Read the model definition and answer for the solid it produces. Units are mm, in the model's axes. Face numbers are marked on the shaded views. A direction names the side the tool comes from. Give positions to 0.01 mm unless a question says otherwise; leave off trailing zeros. Write each loop counter-clockwise with the first axis right and the second up, starting at its lowest first coordinate (ties: lowest second). Pieces come first, ordered by that corner, then holes. Notation, with made-up numbers: (-16, 70) -> (1, 70) arc R9 ccw to (1, 80) -> close; hole circle Ø1 at (34, 2.25). An arc over 180 degrees is marked (long way). Use a Markdown table: item, result.
from build123d import *

# Parameters (mm, degrees)
PAD002_DEPTH    = 5.55
POCKET001_DEPTH = 0.5
POCKET002_DEPTH = 0.5
PAD003_DEPTH    = 2.5
PAD001_DEPTH    = 9
SKETCH_R        = 9
PAD_DEPTH       = 11.8
SKETCH001_R     = 11.05
POCKET_DEPTH    = 10
SKETCH010_R     = 1.55
POCKET003_DEPTH = 5
FILLET_R        = 1.8
SKETCH012_W     = 10.3286741025
SKETCH012_H     = 11.8
PAD004_DEPTH    = 2.4
SKETCH011_R     = 2.1
POCKET004_DEPTH = 6.4010000001
POCKET005_DEPTH = 4
FILLET001_R     = 2
FILLET002_R     = 2
FILLET003_R     = 2


with BuildPart() as pad003:
    # Sketch004 → Pad002 (new body)
    with BuildSketch(Plane.XY.offset(2.225)):
        Polygon((-11.1717282118, -2.7499991288), (-7.9674332118, -8.3000008712), (-8.4004459137, -8.5500008712), (-11.6047409137, -2.9999991288), align=None)
    extrude(amount=PAD002_DEPTH)

    # Sketch006 → Pocket001 (cut)
    with BuildSketch(Plane(origin=(-9.5695807118, -5.525, 2.225), x_dir=(-0.5, 0.8660254038, 0), z_dir=(0.8660254038, 0.5, 0))):
        Polygon((-3.204295, 2.7750019602), (-1.6021491347, 5.55), (-3.204295, 5.55), align=None)
        Polygon((1.6021478772, 0), (3.204295, 0), (3.204295, 2.7750019602), align=None)
    extrude(amount=-POCKET001_DEPTH, mode=Mode.SUBTRACT)

    # Sketch008 → Pocket002 (cut)
    with BuildSketch(Plane(origin=(-9.5695807118, -5.525, 2.225), x_dir=(-0.5, 0.8660254038, 0), z_dir=(0.8660254038, 0.5, 0))):
        Polygon((1.6021478772, 5.5500030493), (3.204295, 5.5500030493), (3.204295, 2.7750019602), align=None)
        Polygon((-1.6021478772, 0), (-3.2042957545, 0), (-3.2042957545, 2.7750015246), align=None)
    extrude(amount=-POCKET002_DEPTH, mode=Mode.SUBTRACT)

    # Sketch009 → Pad003 (new body, symmetric)
    with BuildSketch(Plane(origin=(-9.5695807118, -5.525, 2.225), x_dir=(-0.5, 0.8660254038, 0), z_dir=(0.8660254038, 0.5, 0))):
        Polygon((1.6021491347, -7.4054e-06), (3.2042982695, 2.7749962973), (1.6021491347, 5.55), (-1.6021491347, 5.55), (-3.2042982695, 2.7749962973), (-1.6021491347, -7.4054e-06), align=None)
    extrude(amount=PAD003_DEPTH, both=True)


with BuildPart() as pad001:
    # Sketch003 → Pad001 (new body)
    with BuildSketch(Plane.XY):
        with BuildLine():
            ThreePointArc((-10.9554657182, -1.442314424), (-9.5695807118, -5.525), (-6.7268137905, -8.7665544102))
            Line((-10.3793823646, -13.526674452), (-6.7268137905, -8.7665544102))
            ThreePointArc((-16.9041348864, -2.2254715773), (-14.7657331345, -8.525), (-10.3793823646, -13.526674452))
            Line((-10.9554657182, -1.442314424), (-16.9041348864, -2.2254715773))
        make_face()
    extrude(amount=PAD001_DEPTH)


with BuildPart() as fillet003:
    # Sketch → Pad (new body)
    with BuildSketch(Plane.XY):
        with BuildLine():
            Line((-23, 11.5), (23, 11.5))
            Line((23, 11.5), (23, 7.5))
            Line((23, 7.5), (15, 7.5))
            Line((12.6713258975, 7.5), (15, 7.5))
            Line((12.6713258975, 4.8), (12.6713258975, 7.5))
            ThreePointArc((-12.6713258975, 4.8), (0, -13.55), (12.6713258975, 4.8))
            Line((-12.6713258975, 7.5), (-12.6713258975, 4.8))
            Line((-15, 7.5), (-12.6713258975, 7.5))
            Line((-15, 7.5), (-23, 7.5))
            Line((-23, 7.5), (-23, 11.5))
        make_face()
        Circle(SKETCH_R, mode=Mode.SUBTRACT)
    extrude(amount=PAD_DEPTH)

    # Sketch001 → Pocket (cut)
    with BuildSketch(Plane.XY.offset(11.8)):
        Circle(SKETCH001_R)
    extrude(amount=-POCKET_DEPTH, mode=Mode.SUBTRACT)

    # Fusion: union Pad001
    add(pad001.part)

    # Cut: cut Pad003
    add(pad003.part, mode=Mode.SUBTRACT)

    # Sketch010 → Pocket003 (cut)
    with BuildSketch(Plane(origin=(-11.7346442213, -6.775, 0), x_dir=(-0.5, 0.8660254038, 0), z_dir=(0.8660254038, 0.5, 0))):
        with Locations((0, 4.9999962973)):
            Circle(SKETCH010_R)
    extrude(amount=-POCKET003_DEPTH, mode=Mode.SUBTRACT)

    # Fillet
    fillet_edges = [fillet003.edges().sort_by_distance(p)[0] for p in [
        (-12.671326, 4.8, 5.9),
        (12.671326, 4.8, 5.9),
    ]]
    fillet(fillet_edges, radius=FILLET_R)

    # Sketch012 → Pad004 (new body)
    with BuildSketch(Plane.XZ.offset(-7.5)):
        with Locations((-17.8356629487, 5.9)):
            Rectangle(SKETCH012_W, SKETCH012_H)
        with Locations((17.8356629487, 5.9)):
            Rectangle(SKETCH012_W, SKETCH012_H)
    extrude(amount=PAD004_DEPTH)

    # Sketch011 → Pocket004 (cut, through all)
    with BuildSketch(Plane.XZ.offset(-5.1)):
        with Locations((-18.5, 5.9)):
            Circle(SKETCH011_R)
        with Locations((18.5, 5.9)):
            Circle(SKETCH011_R)
    extrude(amount=-POCKET004_DEPTH, mode=Mode.SUBTRACT)

    # Sketch013 → Pocket005 (cut)
    with BuildSketch(Plane.XZ.offset(-5.1)):
        Polygon((-14.4296806022, 5.9), (-16.4648403011, 9.425), (-20.5351596989, 9.425), (-22.5703193978, 5.9), (-20.5351596989, 2.375), (-16.4648403011, 2.375), align=None)
        Polygon((22.5703193978, 5.9), (20.5351596989, 9.425), (16.4648403011, 9.425), (14.4296806022, 5.9), (16.4648403011, 2.375), (20.5351596989, 2.375), align=None)
    extrude(amount=-POCKET005_DEPTH, mode=Mode.SUBTRACT)

    # Fillet001
    fillet001_edges = [fillet003.edges().sort_by_distance(p)[0] for p in [
        (-23, 6.3, 0),
        (-23, 9.5, 0),
        (-23, 9.5, 11.8),
        (-23, 6.3, 11.8),
        (23, 6.3, 0),
        (23, 9.5, 0),
        (23, 9.5, 11.8),
        (23, 6.3, 11.8),
    ]]
    fillet(fillet001_edges, radius=FILLET001_R)

    # Fillet002
    fillet002_edges = [fillet003.edges().sort_by_distance(p)[0] for p in [
        (-8.248717, -10.749938, 4.5),
        (-13.434078, -1.76863, 4.5),
    ]]
    fillet(fillet002_edges, radius=FILLET002_R)

    # Fillet003
    fillet003_edges = [fillet003.edges().sort_by_distance(p)[0] for p in [
        (-10.379382, -13.526674, 4.5),
        (-16.904135, -2.225472, 4.5),
    ]]
    fillet(fillet003_edges, radius=FILLET003_R)


solid = fillet003.part
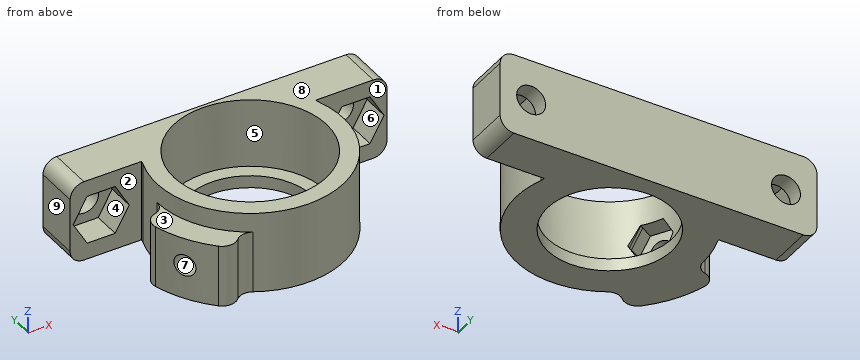
Item 1: A cutting plane is placed at C-C (x = 10). Give the vertices of the cut face in (y, z).
Return value:
| item | result |
|---|---|
| outline | (-9.14, 0) -> (11.5, 0) -> (11.5, 11.8) -> (4.7, 11.8) -> (4.7, 1.8) -> (-4.7, 1.8) -> (-4.7, 11.8) -> (-9.14, 11.8) -> close |
Item 2: A tool of negligible diameter and unlimited length cuts with its end or side. For the marked faces 1, 2, 3, 4 and 5, from which of +Z, -Z, +X, -X, +Y, -Y can it reach the whole face along a straight path? Write none if from no direction.
Return value:
| item | result |
|---|---|
| face 1 | +Z, -Z, +X |
| face 2 | +Z, -Z, -X |
| face 3 | +Z, -X, -Y |
| face 4 | none |
| face 5 | +Z |
Item 3: For a pull along Z with two mould halves and no side action, classify the marked faces 6, 7, 8 and 9 as +Z half, -Z half, draft (parallel to the pull), parting line (faces both ways), or undercut.
Return value:
| item | result |
|---|---|
| face 6 | undercut |
| face 7 | undercut |
| face 8 | +Z half |
| face 9 | draft |
Item 4: A cutting plane is placed at A-A (x = 0). Give the vertices of the cut face in (y, z).
Return value:
| item | result |
|---|---|
| outline | (-13.55, 0) -> (-9, 0) -> (-9, 1.8) -> (-11.05, 1.8) -> (-11.05, 11.8) -> (-13.55, 11.8) -> close; (9, 0) -> (11.5, 0) -> (11.5, 11.8) -> (11.05, 11.8) -> (11.05, 1.8) -> (9, 1.8) -> close |
Item 5: Each of these flat-tipped pins is pushed along its axis until it touches: P1, Ø5, axis at x = 19.5, z = 3.5, coming from the -Y side; P2, Ø1, axis at x = -13, z = 6, coming from the -Y side; P3, Ø3.5, axis at x = 17, z = 6.5, coming from the -Y side; P4, Ø1, axis at x = 14.5, y = 3, coming from the -Z side. Where does it stop, or does it pass through?
Return value:
| item | result |
|---|---|
| P1 | y = 5.1 |
| P2 | y = -11.6 |
| P3 | y = 9.1 |
| P4 | through |
Item 6: Straight lines are drawn through the part: line 1 along Y through (x, z) = (0, 6.25); line 2 along Z through (x, y) = (-19.5, 6.75) (3 decimals); line 3 along Y through (x, z) = (0, 0.8). For each, find the intervals that lie inside material, in ascending order. Write a range as [from, to].
Return value:
| item | result |
|---|---|
| line 1 | [-13.55, -11.05], [11.05, 11.5] |
| line 2 | [0, 2.375], [9.425, 11.8] |
| line 3 | [-13.55, -9], [9, 11.5] |
Item 7: A cutting plane is placed at B-B (y = 2). Give the vertices of the cut face in (x, z).
Return value:
| item | result |
|---|---|
| outline | (-13.4, 0) -> (-8.77, 0) -> (-8.77, 1.8) -> (-10.87, 1.8) -> (-10.87, 11.8) -> (-13.4, 11.8) -> close; (8.77, 0) -> (13.4, 0) -> (13.4, 11.8) -> (10.87, 11.8) -> (10.87, 1.8) -> (8.77, 1.8) -> close |
